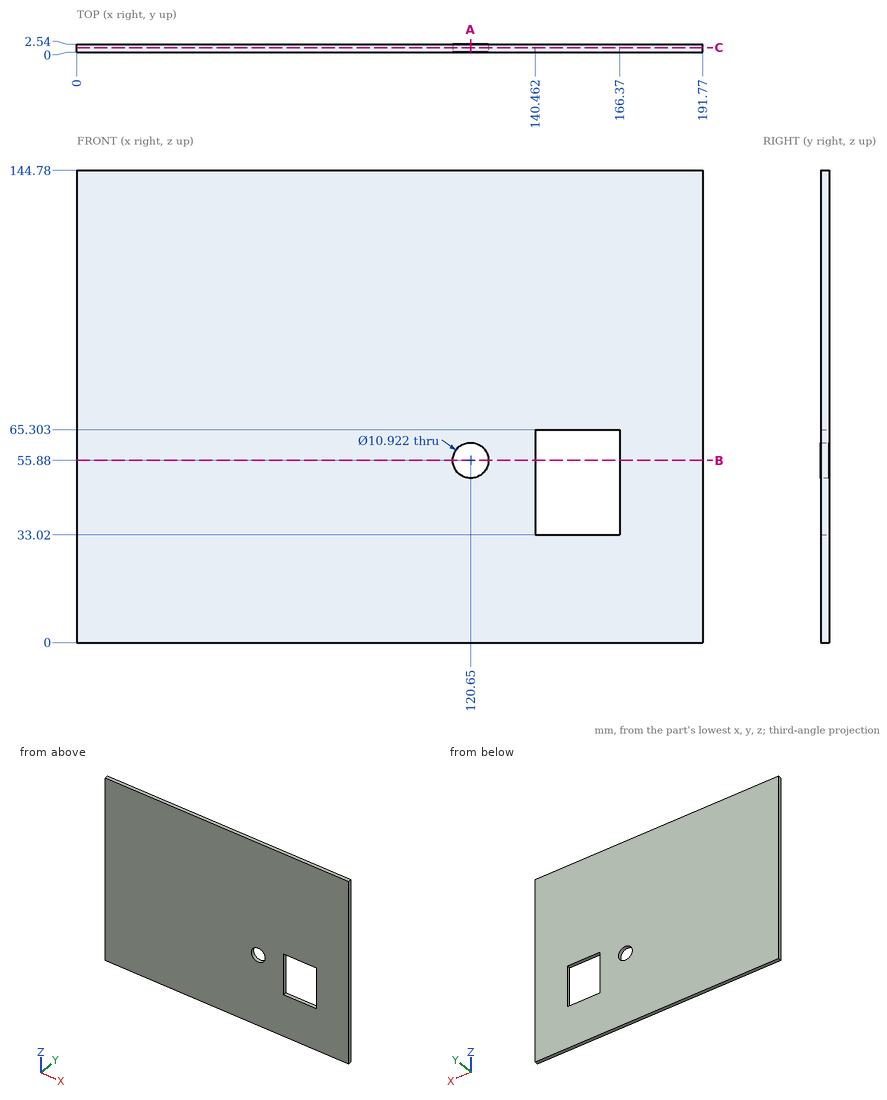
Part print with two shaded views. Sizes in mm from the minimum x, y, z corner. Round coordinates to 2 decimals unless told otherwise and drop trailing zeros. Write each loop counter-clockwise with the first axis right and the second up, starting at its lowest first coordinate (ties: lowest second). Pieces come first, ordered by that corner, then holes. Notation, with made-up numbers: M 64.25,32 L 94.25,32 A10 ccw 94.25,46 Z; hole C -11,54 d4. An arc over 180 degrees is marked long. Use CSV: the item, a comma, the result in double quotes.
1. Saw through at B-B (z = 55.88). Give the cut face in (x, y).
Reply:
outline,"M 0,0 L 115.19,0 L 115.19,2.54 L 0,2.54 Z; M 126.11,0 L 140.46,0 L 140.46,2.54 L 126.11,2.54 Z; M 166.37,0 L 191.77,0 L 191.77,2.54 L 166.37,2.54 Z"
2. Saw through at A-A (x = 120.65). Give the cut face in (y, z), plus the area to 3 significant figures.
Reply:
outline,"M 0,0 L 2.54,0 L 2.54,50.42 L 0,50.42 Z; M 0,61.34 L 2.54,61.34 L 2.54,144.78 L 0,144.78 Z"
area,"340 mm²"
3. Saw through at C-C (y = 1.4). Give the cut face in (x, z), plus the area to 3 significant figures.
Reply:
outline,"M 0,0 L 191.77,0 L 191.77,144.78 L 0,144.78 Z; hole C 120.65,55.88 d10.92; hole M 140.46,33.02 L 166.37,33.02 L 166.37,65.3 L 140.46,65.3 Z"
area,"26,800 mm²"
4. Wall check: probe 1 along X at (y, z) = (0.65, 55.88); probe 2 along Z at (x, y) = (147.5, 2.1); probe 3 along X at (y, z) = (2.1, 39). Give the ranges that are in metal, low to high. Write a range as from..to.
Reply:
probe 1,"x = 0..115.19, 126.11..140.46, 166.37..191.77"
probe 2,"z = 0..33.02, 65.3..144.78"
probe 3,"x = 0..140.46, 166.37..191.77"
